Geometry: final body of the model. Coordinates: model frame, mm. Give positions to 0.01 mm unless a question says otherwise; leave off trailing zeros. Write each loop counter-clockwise with the first axis right and the second up, starting at its lowest first coordinate (ties: lowest second). Pieces come first, ordered by that corner, then holes.
Q1. Cut plane C-C on z = 54. Return the cut outline in (x, y).
Q2. Pin query (flat end, axial travel): pin 1 (6 mm diameter, centred on y = 6, z = 206.5, fed in from +X); pin 2 (10 mm diameter, centred on x = 5.5, z = 52, fed in from -Y). Return the tip coordinate at first contact, or that it passes through.
Q3. Cut plane A-A on x = 0. Return the cut outline in (y, z), plus the area to 3 significant figures.
Q4. Line query: L1, parallel to Z at x = 3.5, y = -15.5; L2, parallel to Z at x = 12.5, y = -2; L3, parallel to Y at x = -3, z = 29. Output: solid intervals per line, ascending.
Q5. Draft query along Y for faces 1 (the face through (0, 0, 0)), 2 (the face through (-0.867, -3.905, 107.474)). Return one class per face: pulls with the +Y half, pulls with the -Y half, needs draft (parallel to the pull), parting line crosses it, or undercut.
```python
from build123d import *

# Parameters (mm, degrees)
SKETCH1_R           = 23.85
BOSS_EXTRUDE1_DEPTH = 230
SKETCH2_OUTSIDE_W   = 97.638
SKETCH2_OUTSIDE_H   = 97.638
SKETCH2_OUTSIDE_R   = 4
CUT_EXTRUDE1_DEPTH  = 218


with BuildPart() as part:
    # Sketch1 → Boss-Extrude1 (new body)
    with BuildSketch(Plane.XY):
        Circle(SKETCH1_R)
    extrude(amount=BOSS_EXTRUDE1_DEPTH)

    # Sketch2 outside → Cut-Extrude1 (cut)
    with BuildSketch(Plane.XY):
        Rectangle(SKETCH2_OUTSIDE_W, SKETCH2_OUTSIDE_H)
        Circle(SKETCH2_OUTSIDE_R, mode=Mode.SUBTRACT)
    extrude(amount=CUT_EXTRUDE1_DEPTH, mode=Mode.SUBTRACT)

    # Sketch5 → Cut-Revolve1 (revolve, cut)
    with BuildSketch(Plane(origin=(0, 0, 0), x_dir=(1, 0, 0), z_dir=(0, 1, 0))):
        Polygon((4, -218), (23.85, -225.22480915), (23.85, -218), align=None)
    revolve(axis=Axis((0, 0, 0), (0, 0, 1)), mode=Mode.SUBTRACT)


solid = part.part
```
Data:
1. outline: circle Ø8 at (0, 0)
2. pin 1: stops at x = 2.65
2. pin 2: stops at y = -3.97
3. outline: (-23.85, 225.22) - (-4, 218) - (-4, 0) - (4, 0) - (4, 218) - (23.85, 225.22) - (23.85, 230) - (-23.85, 230) - close
3. area: 2,170 mm2
4. L1: z = 222.33 to 230
4. L2: z = 221.15 to 230
4. L3: y = -2.65 to 2.65
5. face 1: needs draft
5. face 2: parting line crosses it
